Input: dimensioned drawing with shaded views. Units: mm. Origin: part minimum x, y, z. Coordinates: 2 decimals unless noted, no trailing zeros. Loops run counter-clockwise (first coordinate to the right, second up) from the corner with the lowest first, then second, coordinate; pieces in that order, holes last.
Item 1: Section D-D on z = 8.5. Return loops of the section in (x, y) (1 decimal), and give its area (3 significant figures).
Item 2: Section B-B on x = 9. Return loops of the section in (y, z).
Item 3: Pull-direction query (X, two-part tool) for the marked faces 1, 2 and 3; classes: released by +X, released by -X, zero draft, split by the parting line, or undercut.
Item 4: Contact query for flat-ended pins moving along their axis: P1, Ø5, axis at x = 18, z = 11, coming from the +Y side; P2, Ø2.5, axis at x = 19.13, z = 19.13, coming from the +Y side. Output: stop coordinate, or through.
Item 5: Ray query, line 1 along Z through (x, y) = (11, 1.45); line 2 along X through (y, z) = (1.15, 10.75); line 3 along X through (y, z) = (0.4, 3) (1 decimal). Return the intervals inside material, ascending.
Item 6: Section C-C on x = 3.25. Return loops of the section in (y, z).
Item 7: Section A-A on z = 12. Return loops of the section in (x, y) (1 decimal).
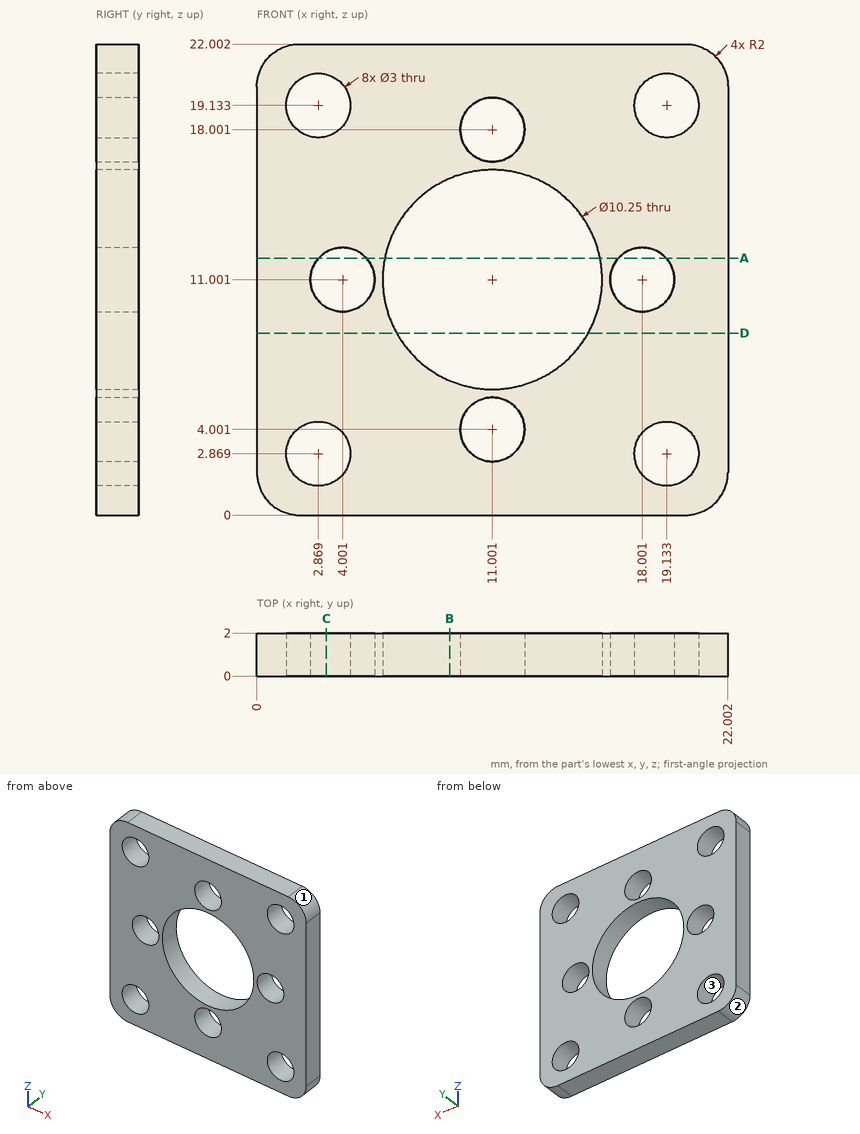
Results found:
1. outline: (0, 0) - (6.5, 0) - (6.5, 2) - (0, 2) - close; (15.5, 0) - (22, 0) - (22, 2) - (15.5, 2) - close
1. area: 26.1 mm2
2. outline: (0, 0) - (2, 0) - (2, 6.28) - (0, 6.28) - close; (0, 15.72) - (2, 15.72) - (2, 22) - (0, 22) - close
3. face 1: released by +X
3. face 2: released by -X
3. face 3: undercut
4. P1: stops at y = 2
4. P2: passes through
5. line 1: z = 0 to 2.5, 5.5 to 5.88, 16.13 to 16.5, 19.5 to 22
5. line 2: x = 0 to 2.52, 5.48 to 5.88, 16.12 to 16.52, 19.48 to 22
5. line 3: x = 0 to 1.4, 4.4 to 9.9, 12.1 to 17.6, 20.6 to 22
6. outline: (0, 0) - (2, 0) - (2, 1.42) - (0, 1.42) - close; (0, 4.32) - (2, 4.32) - (2, 9.7) - (0, 9.7) - close; (0, 12.3) - (2, 12.3) - (2, 17.68) - (0, 17.68) - close; (0, 20.58) - (2, 20.58) - (2, 22) - (0, 22) - close
7. outline: (0, 0) - (2.9, 0) - (2.9, 2) - (0, 2) - close; (5.1, 0) - (6, 0) - (6, 2) - (5.1, 2) - close; (16, 0) - (16.9, 0) - (16.9, 2) - (16, 2) - close; (19.1, 0) - (22, 0) - (22, 2) - (19.1, 2) - close
